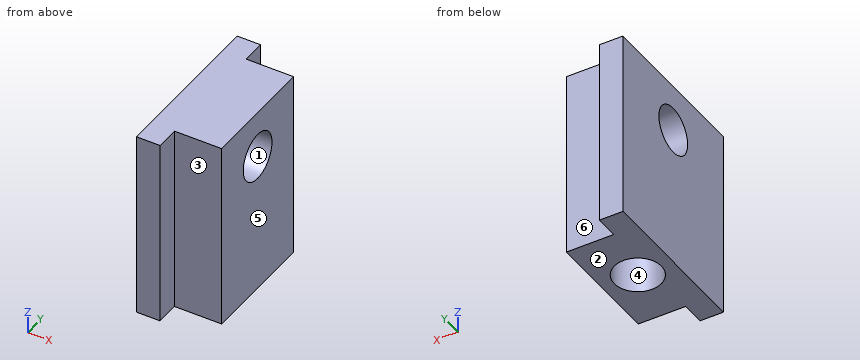
```python
from build123d import *

# Parameters (mm, degrees)
BOSS_EXTRUDE1_DEPTH             = 25.4
SKETCH3_R                       = 3.175
CUT_EXTRUDE1_DEPTH              = 36.06902123
F_1_4_0_25_DIAMETER_HOLE1_D     = 6.35
F_1_4_0_25_DIAMETER_HOLE1_DEPTH = 12.7
F_1_4_0_25_DIAMETER_HOLE1_TIP   = 1.907732465


with BuildPart() as part:
    # Sketch1 → Boss-Extrude1 (new body)
    with BuildSketch(Plane.XY):
        Polygon((0, 0), (3.175, 0), (3.175, 3.175), (9.525, 3.175), (9.525, 19.05), (3.175, 19.05), (3.175, 22.225), (0, 22.225), align=None)
    extrude(amount=BOSS_EXTRUDE1_DEPTH)

    # Sketch3 → Cut-Extrude1 (cut, through all)
    with BuildSketch(Plane(origin=(9.525, 0, 0), x_dir=(0, 0, -1), z_dir=(1, 0, 0))):
        with Locations((-19.05, 11.1125)):
            Circle(SKETCH3_R)
    extrude(amount=-CUT_EXTRUDE1_DEPTH, mode=Mode.SUBTRACT)

    # 1/4 (0.25) Diameter Hole1
    with Locations(Plane(origin=(0, 0, 0), x_dir=(-1, 0, 0), z_dir=(0, 0, -1))):
        with Locations((-4.7625, 11.1125)):
            Hole(F_1_4_0_25_DIAMETER_HOLE1_D / 2, depth=F_1_4_0_25_DIAMETER_HOLE1_DEPTH)
            with Locations((0, 0, -(F_1_4_0_25_DIAMETER_HOLE1_DEPTH + F_1_4_0_25_DIAMETER_HOLE1_TIP / 2))):  # 118° drill point
                Cone(0, F_1_4_0_25_DIAMETER_HOLE1_D / 2, F_1_4_0_25_DIAMETER_HOLE1_TIP, mode=Mode.SUBTRACT)


solid = part.part
```
Can you work these out from the model? Positions are in its coordinate system, mm. Face numbers are marked on the shaded views. A direction names the side the tool comes from. Coordinates: 2 decimals unless noted, no trailing zeros. Loops run counter-clockwise (first coordinate to the right, second up) from the corner with the lowest first, then second, coordinate; pieces in that order, holes last.
Item 1: Which directions (+Z, -Z, +X, -X, +Y, -Y) give clear straight access to the entire face, cutting with the end or side of a thin tool? Please do the marked faces 4, 5 and 6.
Answers below:
face 4: -Z
face 5: +Z, -Z, +X, +Y, -Y
face 6: +Z, -Z, +X, +Y
Item 2: I'm going to push flat-ended pins straight in: pin 1 (4 mm diameter, centred on y = 11.11, z = 19.05, fed in from +X); pin 2 (3.5 mm diameter, centred on y = 20.5, z = 12.5, fed in from +X) (3 decimals); pin 3 (1.9 mm diameter, centred on x = 7, z = 8, fed in from +Y); pin 4 (1 mm diameter, centred on y = 2.5, z = 15.5, fed in from +X) (3 decimals). Where does each tip first touch, or does it pass through?
Answers below:
pin 1: passes through
pin 2: stops at x = 9.525
pin 3: stops at y = 19.05
pin 4: stops at x = 3.175
Item 3: If we mould it in two halves opening along Z, with no side actions, what happens to the marked faces 1, 2 and 3? For each: released by +Z, released by -Z, zero draft, split by the parting line, or undercut.
Answers below:
face 1: undercut
face 2: released by -Z
face 3: zero draft
Item 4: Suppose I cut it at D-D (y = 19.75). Please give me the cut outline in (x, z) (3 decimals).
Answers below:
outline: (0, 0) - (3.175, 0) - (3.175, 25.4) - (0, 25.4) - close
Item 5: Please list where these lines run through material, in increasing order: L1, parallel to Y at x = 2.75, z = 19.05 (1 decimal); L2, parallel to Y at x = 3.25, z = 15.5 (3 decimals); L3, parallel to Z at x = 4.75, y = 13.5.
Answers below:
L1: y = 0 to 7.9, 14.3 to 22.2
L2: y = 3.175 to 19.05
L3: z = 13.17 to 16.96, 21.14 to 25.4
